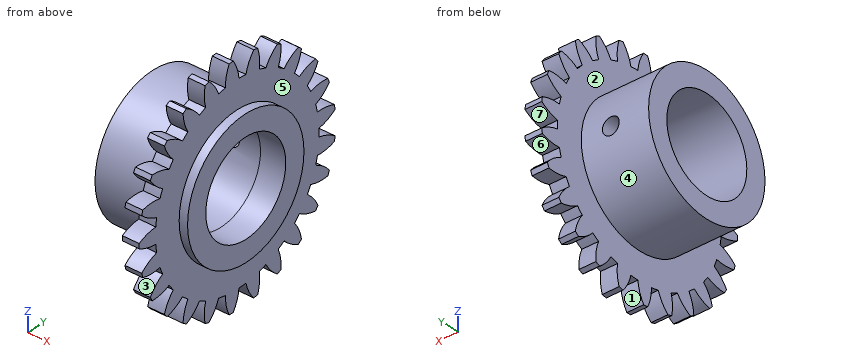
from build123d import *

# Parameters (mm, degrees)
BASPROSKE_W        = 2
BASPROSKE_H        = 13.5
TOOTHCUT_DEPTH     = 20.19635382
TEETHCUTS_COUNT    = 25
TEETHCUTS_ANGLE    = 345.6
BORSKE_R           = 5.5
BORE_DEPTH         = 50.0000508
BOSS_EXTRU_1_START = 1
ESQUISSE1_R        = 8
ESQUISSE1_R_2      = 5.5
BOSS_EXTRU_1_DEPTH = 1
ESQUISSE2_R        = 8
ESQUISSE2_R_2      = 5.5
BOSS_EXTRU_2_DEPTH = 8
ESQUISSE4_W        = 1
ESQUISSE4_H        = 13.425711508


with BuildPart() as part:
    # BasProSke → Base-Revolve (revolve)
    with BuildSketch(Plane(origin=(0, 0, 0), x_dir=(1, 0, 0), z_dir=(0, 1, 0)), mode=Mode.PRIVATE) as base_revolve_sk:
        with Locations((1, 6.75)):
            Rectangle(BASPROSKE_W, BASPROSKE_H)
    revolve(base_revolve_sk.sketch.rotate(Axis((-10, 0, 0), (1, 0, 0)), 180), axis=Axis((-10, 0, 0), (1, 0, 0)))

    # TooCutSke → ToothCut (cut, through all)
    with BuildSketch(Plane(origin=(0, 0, 0), x_dir=(0, 0, -1), z_dir=(1, 0, 0))):
        with BuildLine():
            ThreePointArc((0.480087995, 11.238750665), (0, 11.249), (-0.480087995, 11.238750665))
            ThreePointArc((-0.480087995, 11.238750665), (-0.821124963, 12.40220054), (-1.432168974, 13.449361962))
            ThreePointArc((-1.432168974, 13.449361962), (0, 13.5254), (1.432168974, 13.449361962))
            ThreePointArc((1.432168974, 13.449361962), (0.821124963, 12.40220054), (0.480087995, 11.238750665))
        make_face()
    toothcut = extrude(amount=TOOTHCUT_DEPTH, mode=Mode.SUBTRACT)

    # TeethCuts: ToothCut ×25 about axis
    teethcuts_axis = Axis((-10, 0, 0), (1, 0, 0))
    for i in range(1, TEETHCUTS_COUNT):
        add(toothcut.rotate(teethcuts_axis, i * TEETHCUTS_ANGLE / (TEETHCUTS_COUNT - 1)), mode=Mode.SUBTRACT)

    # BorSke → Bore (cut, symmetric)
    with BuildSketch(Plane(origin=(0, 0, 0), x_dir=(0, 0, -1), z_dir=(1, 0, 0))):
        with Locations(Location((0, 0, 0), (0, 0, 180))):
            Circle(BORSKE_R)
    extrude(amount=BORE_DEPTH, both=True, mode=Mode.SUBTRACT)

    # Esquisse1 → Boss.-Extru.1 (add)
    with BuildSketch(Plane(origin=(2, 0, 0), x_dir=(0, 0, -1), z_dir=(1, 0, 0)).offset(BOSS_EXTRU_1_START)):
        with Locations(Location((0, 0, 0), (0, 0, 180))):
            Circle(ESQUISSE1_R)
        Circle(ESQUISSE1_R_2, mode=Mode.SUBTRACT)
    extrude(amount=-BOSS_EXTRU_1_DEPTH)

    # Esquisse2 → Boss.-Extru.2 (add)
    with BuildSketch(Plane.ZY):
        Circle(ESQUISSE2_R)
        Circle(ESQUISSE2_R_2, mode=Mode.SUBTRACT)
    extrude(amount=BOSS_EXTRU_2_DEPTH)

    # Esquisse4 → Diamètre du perçage Ø2.0 (2)1 (revolve, cut)
    with BuildSketch(Plane(origin=(-3.5, 0, 0), x_dir=(0, 0, -1), z_dir=(1, 0, 0))):
        with Locations((0.5, 6.712855754)):
            Rectangle(ESQUISSE4_W, ESQUISSE4_H)
    revolve(axis=Axis((-3.5, -6.35, 0), (0, 1, 0)), mode=Mode.SUBTRACT)


solid = part.part
Can you work these out from the model? Positions are in its coordinate system, mm. Face numbers are marked on the shaded views. A direction names the side the tool comes from. Round coordinates to 2 decimals unless told otherwise and drop trailing zeros. Order: outer loops, then holes, each group sorted by start corner. A loop starts at its lowest first (then second) coordinate and runs counter-clockwise, first axis right, second up. Notation, with made-up numbers: (65, -12.5) -> (87, -12.5) arc R19 ccw to (87, 7.5) -> close; hole circle Ø3 at (-1, 29). An arc over 180 degrees is marked (long way). Write each question's results on one line, items separated by ' | '. Start each with the question number.
Item 1: If we section it at A-A, the plane y = -3.25: Write out the boundary of the cut face in (x, z).
Item 2: If we section it at C-C, the plane x = -3.5: Write out the boundary of the cut face in (y, z).
Item 3: Please list where these lines run through material, in increasing order: L1, parallel to Y at x = 0.85, z = 0; L2, parallel to Y at x = -2.25, z = 0; L3, parallel to X at y = 6.65, z = 0.
Item 4: If we section it at B-B, the plane x = -5: Write out the boundary of the cut face in (y, z), then the cut area to 3 significant figures.
Item 5: Thinking about a two-plate mould opening in Z: for the marked faces 1, 2, 3 and 4, which applies, +Z half, -Z half, draft (parallel to the pull), parting line (faces both ways), or undercut?
Item 6: Which directions (+Z, -Z, +X, -X, +Y, -Y) give clear straight access to the entire face, cutting with the end or side of a thin tool? Please do the marked faces 5, 6 and 7.
Item 7: Will these pins go through, and if not, where does the flat tip stop? pin 1 (2.5 mm diameter, centred on x = -3.5, z = 0, fed in from -Y); pin 2 (5 mm diameter, centred on x = -1, z = -4.5, fed in from -Y); pin 3 (2 mm diameter, centred on x = -3.5, y = -7.5, fed in from -Z).
Results:
1) outline: (-8, -7.31) -> (0, -7.31) -> (0, -12.2) -> (2, -12.2) -> (2, -7.31) -> (3, -7.31) -> (3, -4.44) -> (-8, -4.44) -> close; (-8, 4.44) -> (3, 4.44) -> (3, 7.31) -> (2, 7.31) -> (2, 12.2) -> (0, 12.2) -> (0, 7.31) -> (-8, 7.31) -> close
2) outline: (5.41, -1) arc R5.5 cw (long way) to (5.41, 1) -> (7.94, 1) arc R8 ccw (long way) to (7.94, -1) -> close
3) L1: y = -13.5 to -5.5, 5.5 to 11.25 | L2: y = -8 to -5.5, 5.5 to 8 | L3: x = -8 to -4.5, -2.5 to 3
4) outline: circle Ø16 at (0, 0); hole circle Ø11 at (0, 0) | area: 106 mm2
5) face 1: -Z half | face 2: draft | face 3: undercut | face 4: parting line
6) face 5: +X | face 6: +X, -X | face 7: +X, -X, +Y
7) pin 1: stops at y = -8 | pin 2: stops at y = -13.14 | pin 3: stops at z = -4.66
